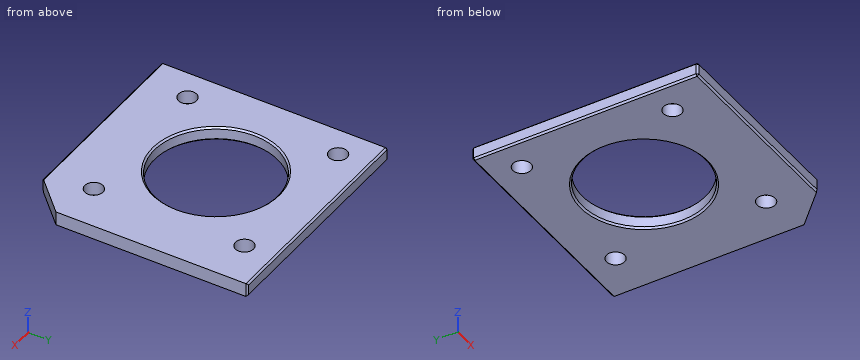
from build123d import *

# Parameters (mm, degrees)
ESQUISSE1_W        = 66
ESQUISSE1_H        = 66
ESQUISSE1_R        = 18
BOSS_EXTRU_1_DEPTH = 4
CHANFREIN1_SIZE    = 10
CHANFREIN2_SIZE    = 0.5
D_GAGEMENT_M51_D   = 5.3


with BuildPart() as part:
    # Esquisse1 → Boss.-Extru.1 (new body)
    with BuildSketch(Plane.XY):
        Rectangle(ESQUISSE1_W, ESQUISSE1_H)
        with Locations((-2, 2)):
            Circle(ESQUISSE1_R, mode=Mode.SUBTRACT)
    extrude(amount=BOSS_EXTRU_1_DEPTH)

    # Chanfrein1
    chanfrein1_edges = [part.edges().sort_by_distance(p)[0] for p in [
        (33, -33, 2),
    ]]
    chamfer(chanfrein1_edges, length=CHANFREIN1_SIZE)

    # Chanfrein2
    chanfrein2_edges = [part.edges().sort_by_distance(p)[0] for p in [
        (-33, 0, 4),
        (-20, 2, 0),
        (-20, 2, 4),
        (-5, -33, 4),
        (-5, -33, 0),
        (-33, 0, 0),
        (0, 33, 0),
        (0, 33, 4),
        (-33, -33, 2),
        (-33, 33, 2),
        (33, 33, 2),
    ]]
    chamfer(chanfrein2_edges, length=CHANFREIN2_SIZE)

    # Dégagement M51 (through all)
    with Locations(Plane.XY.offset(4)):
        with Locations((-24, 24), (20, 24), (20, -20), (-24, -20), (-162.098619818, 40.106243937), (-166.138996893, 40.106243937)):
            Hole(D_GAGEMENT_M51_D / 2)


solid = part.part
Design review of the part built by this model. Coordinates are the model's own, in mm. Coordinates: 2 decimals unless noted, no trailing zeros. Loops run counter-clockwise (first coordinate to the right, second up) from the corner with the lowest first, then second, coordinate; pieces in that order, holes last. Notation, with made-up numbers: (-9, 26) -> (2, 26) arc R19 cw to (2, 44) -> close; hole circle Ø6 at (26.25, 84). An arc over 180 degrees is marked (long way). Use a Markdown table: item, result. Add a question column.
Item 1: We need section A-A, the plane z = 1.9. Write out the cut boundary in (x, y).
Item 2: We need section C-C, the plane x = -24. Write out the cut boundary in (y, z), and give its area (3 significant figures).
Item 3: We need section B-B, the plane y = 2. Write out the cut boundary in (x, z).
Item 4: Wall thickness on L1, parallel to Y at x = 20, z = 3; L2, parallel to X at y = 26, z = 1.6; L3, parallel to X at y = -19, z = 0.2: over which ranges is each line inside the solid? List them lowest first. Write a range as from..to.
Item 5: We need section D-D, the plane y = -20. Write out the cut boundary in (x, z).
Numbers:
| question | item | result |
|---|---|---|
| 1 | outline | (-33, -32.5) -> (-32.5, -33) -> (23, -33) -> (33, -23) -> (33, 32.5) -> (32.5, 33) -> (-32.5, 33) -> (-33, 32.5) -> close; hole circle Ø5.3 at (-24, -20); hole circle Ø5.3 at (-24, 24); hole circle Ø36 at (-2, 2); hole circle Ø5.3 at (20, -20); hole circle Ø5.3 at (20, 24) |
| 2 | outline | (-33, 0.5) -> (-32.5, 0) -> (-22.65, 0) -> (-22.65, 4) -> (-32.5, 4) -> (-33, 3.5) -> close; (-17.35, 0) -> (21.35, 0) -> (21.35, 4) -> (-17.35, 4) -> close; (26.65, 0) -> (32.5, 0) -> (33, 0.5) -> (33, 3.5) -> (32.5, 4) -> (26.65, 4) -> close |
| 2 | area | 221 mm^2 |
| 3 | outline | (-33, 0.5) -> (-32.5, 0) -> (-20.5, 0) -> (-20, 0.5) -> (-20, 3.5) -> (-20.5, 4) -> (-32.5, 4) -> (-33, 3.5) -> close; (16, 0.5) -> (16.5, 0) -> (33, 0) -> (33, 4) -> (16.5, 4) -> (16, 3.5) -> close |
| 4 | L1 | y = -33..-22.65, -17.35..21.35, 26.65..33 |
| 4 | L2 | x = -33..-25.74, -22.26..18.26, 21.74..33 |
| 4 | L3 | x = -32.7..-26.45, -21.55..17.55, 22.45..33 |
| 5 | outline | (-33, 0.5) -> (-32.5, 0) -> (-26.65, 0) -> (-26.65, 4) -> (-32.5, 4) -> (-33, 3.5) -> close; (-21.35, 0) -> (17.35, 0) -> (17.35, 4) -> (-21.35, 4) -> close; (22.65, 0) -> (33, 0) -> (33, 4) -> (22.65, 4) -> close |
